```python
from build123d import *

# Parameters (mm, degrees)
SKETCH1_W                           = 14.478
SKETCH1_H                           = 12.7
BOSS_EXTRUDE1_DEPTH                 = 7.493
F_0_80_TAPPED_HOLE1_D               = 1.19126
F_2_CLEARANCE_HOLE1_D               = 2.2606
F_3_64_0_04688_DIAMETER_HOLE1_D     = 1.190752
F_3_64_0_04688_DIAMETER_HOLE1_DEPTH = 4.7625
F_3_64_0_04688_DIAMETER_HOLE1_TIP   = 0.357737992
SKETCH8_W                           = 7.874
SKETCH8_H                           = 12.7
CUT_EXTRUDE1_DEPTH                  = 2.032
FILLET1_R                           = 3.175


with BuildPart() as part:
    # Sketch1 → Boss-Extrude1 (new body)
    with BuildSketch(Plane(origin=(0, 0, 0), x_dir=(1, 0, 0), z_dir=(0, 1, 0))):
        Rectangle(SKETCH1_W, SKETCH1_H)
    extrude(amount=BOSS_EXTRUDE1_DEPTH)

    # #0-80 Tapped Hole1 (through all)
    with Locations(Plane(origin=(0, 7.493, 0), x_dir=(-1, 0, 0), z_dir=(0, 1, 0))):
        with Locations((3, -3.175), (-3, -3.175)):
            Hole(F_0_80_TAPPED_HOLE1_D / 2)

    # #2 Clearance Hole1 (through all)
    with Locations(Plane(origin=(0, 7.493, 0), x_dir=(-1, 0, 0), z_dir=(0, 1, 0))):
        with Locations((5.6515, 3.175), (-5.6515, 3.175)):
            Hole(F_2_CLEARANCE_HOLE1_D / 2)

    # 3/64 (0.04688) Diameter Hole1
    with Locations(Plane(origin=(0, 0, -6.35), x_dir=(-1, 0, 0), z_dir=(0, 0, -1))):
        with Locations((-2.9972, 3.7465), (2.9972, 3.7465)):
            Hole(F_3_64_0_04688_DIAMETER_HOLE1_D / 2, depth=F_3_64_0_04688_DIAMETER_HOLE1_DEPTH)
            with Locations((0, 0, -(F_3_64_0_04688_DIAMETER_HOLE1_DEPTH + F_3_64_0_04688_DIAMETER_HOLE1_TIP / 2))):  # 118° drill point
                Cone(0, F_3_64_0_04688_DIAMETER_HOLE1_D / 2, F_3_64_0_04688_DIAMETER_HOLE1_TIP, mode=Mode.SUBTRACT)

    # Sketch8 → Cut-Extrude1 (cut)
    with BuildSketch(Plane.XZ.offset(-7.493)):
        with Locations((0, 6.35)):
            Rectangle(SKETCH8_W, SKETCH8_H)
    extrude(amount=CUT_EXTRUDE1_DEPTH, mode=Mode.SUBTRACT)

    # Fillet1
    fillet1_edges = [part.edges().sort_by_distance(p)[0] for p in [
        (3.937, 6.477, 0),
        (-3.937, 6.477, 0),
    ]]
    fillet(fillet1_edges, radius=FILLET1_R)


solid = part.part
```
For this review, take the finished solid that the model builds, in its own axes (mm). A direction names the side the tool comes from. Round coordinates to 2 decimals unless told otherwise and drop trailing zeros. Write each loop counter-clockwise with the first axis right and the second up, starting at its lowest first coordinate (ties: lowest second). Pieces come first, ordered by that corner, then holes. Notation, with made-up numbers: (82, -37.75) - (88, -37.75) arc R19 ccw to (88, -32.75) - close; hole circle Ø1 at (53.5, 24.5). An arc over 180 degrees is marked (long way). Put each result on its own line as item: value.
Q1. We need section A-A (z = 4.5). Give the boundary of the cut face in (x, y).
Solved:
outline: (-7.24, 0) - (7.24, 0) - (7.24, 7.49) - (3.94, 7.49) - (3.94, 5.46) - (-3.94, 5.46) - (-3.94, 7.49) - (-7.24, 7.49) - close
Q2. We need section B-B (y = 7.25). Count the separate pieces of the cut face and the enclosed holes in it, and give its area (3 significant figures).
Solved:
separate pieces: 1
enclosed holes: 4
area: 128 mm2
Q3. Insertion check: pin 1 Ø1 at (x, y) = (3, 3.75) entering from -Z; pin 2 Ø1.8 at (x, z) = (-5.65, 3.18) entering from +Y; pin 3 Ø0.5 at (x, y) = (-0.5, 6.5) entering from +Z. Each pin has a flat end and moves straight along its axis. Give the tip position at first contact, or say it passes through.
Solved:
pin 1: stops at z = -1.53
pin 2: passes through
pin 3: stops at z = 0
Q4. Wall thickness on probe 1 along X at (y, z) = (7.25, 1.75); probe 2 along X at (y, z) = (2.75, -3.5); probe 3 along X at (y, z) = (5.5, 2.5): over which ranges is each line inside the solid? List them lowest first.
Solved:
probe 1: x = -7.24 to -3.6, 3.6 to 7.24
probe 2: x = -7.24 to -3.5, -2.5 to 2.5, 3.5 to 7.24
probe 3: x = -7.24 to -6.56, -4.74 to -3.86, 3.86 to 4.74, 6.56 to 7.24
Q5. Mouldability with a two-part tool opening along Z and no side actions: class faces 4 (the face through (-7.239, 4, 0)), 5 (the face through (2.561, 2.861, -2.772)), 6 (the face through (-3.09, 3.71, -1.29)) as released by +Z, released by -Z, zero draft, split by the parting line, or undercut.
Solved:
face 4: zero draft
face 5: undercut
face 6: released by -Z
Q6. Machinability: for faces 1 (the face through (-2.447, 3.518, -3.935)), 2 (the face through (0, 0, 0)), 3 (the face through (-3.937, 6, 5)), which of the approach directions +Z, -Z, +X, -X, +Y, -Y give a long, thin tool a straight path to every point of the face, cutting with its end or side? Answer none if there is none.
Solved:
face 1: -Z
face 2: +Z, -Z, +X, -X, -Y
face 3: +Z, +Y
Q7. We need section C-C (z = 3). Give the boundary of the cut face in (x, y).
Solved:
outline: (-7.24, 0) - (-6.77, 0) - (-6.77, 7.49) - (-7.24, 7.49) - close; (-4.53, 0) - (4.53, 0) - (4.53, 7.49) - (3.93, 7.49) - (3.93, 5.46) - (-3.93, 5.46) - (-3.93, 7.49) - (-4.53, 7.49) - close; (6.77, 0) - (7.24, 0) - (7.24, 7.49) - (6.77, 7.49) - close
